Can you work these out from the model? Positions are in its coordinate system, mm. A direction names the side the tool comes from. Give positions to 0.01 mm unless a question says otherwise; leave off trailing zeros. Write each loop counter-clockwise with the first axis right and the second up, starting at its lowest first coordinate (ties: lowest second). Pieces come first, ordered by that corner, then holes.
Autodesk Inventor part; units mm, degrees
ref_plane "YZ Plane" through (0, 0, 0) normal (1, 0, 0) x (0, 1, 0)
ref_plane "XZ Plane" through (0, 0, 0) normal (0, 1, 0) x (-1, 0, 0)
ref_plane "XY Plane" through (0, 0, 0) normal (0, 0, 1) x (1, 0, 0)
sketch "Sketch1" plane through (0, 0, 0) normal (0, 1, 0) x (-1, 0, 0)
  circle A0 centre (0, 0) radius 13.3
  circle A1 centre (0, 0) radius 15.3
  dimension "d0" = 26.6
  dimension "d1" = 2
extrude "Extrusion1" add sketch "Sketch1" along normal blind 28 contours A0 | A1
sketch "Sketch2" plane through (0, 0, 0) normal (0, -1, 0) x (1, 0, 0)
  circle A0 centre (0, 0) radius 12
  circle A1 centre (0, 0) radius 14
  dimension "d4" = 24
  dimension "d5" = 2
extrude "Extrusion2" add sketch "Sketch2" along normal blind 30.55 contours A0 | A1
sketch "Sketch3" plane through (0, -30.55, 0) normal (0, -1, 0) x (1, 0, 0)
  circle A0 centre (0, 0) radius 3
  dimension "d8" = 6
extrude "Extrusion3" add sketch "Sketch3" along normal blind 2
sketch "Sketch4" plane through (0, 28, 0) normal (0, 1, 0) x (1, 0, 0)
  circle A0 centre (0, 0) radius 2
  dimension "d11" = 4
extrude "Extrusion4" add sketch "Sketch4" along normal blind 8.1
properties part number "Pump"
(1) Imagine slicing it at B-B, the plane z = 0. Write out the boundary of the cut face in (x, y), plus the area to 3 significant figures.
Returned:
outline: (-15.3, 0) - (-14, 0) - (-14, -30.55) - (-3, -30.55) - (-3, -32.55) - (3, -32.55) - (3, -30.55) - (14, -30.55) - (14, 0) - (15.3, 0) - (15.3, 28) - (2, 28) - (2, 36.1) - (-2, 36.1) - (-2, 28) - (-15.3, 28) - close
area: 1,760 mm2
(2) Imagine slicing it at D-D, the plane x = -13. Write out the boundary of the cut face in (y, z).
Returned:
outline: (-30.55, -5.2) - (0, -5.2) - (0, -8.07) - (28, -8.07) - (28, 8.07) - (0, 8.07) - (0, 5.2) - (-30.55, 5.2) - close
(3) Imagine slicing it at A-A, the plane x = 0. Write out the boundary of the cut face in (y, z).
Returned:
outline: (-32.55, -3) - (-30.55, -3) - (-30.55, -14) - (0, -14) - (0, -15.3) - (28, -15.3) - (28, -2) - (36.1, -2) - (36.1, 2) - (28, 2) - (28, 15.3) - (0, 15.3) - (0, 14) - (-30.55, 14) - (-30.55, 3) - (-32.55, 3) - close
(4) Will these pins go through, and if not, where does the flat tip stop? P1, Ø1, axis at x = -5.5, y = 13.5, coming from the +Z side; P2, Ø2, axis at x = -9.5, z = -4.5, coming from the +Y side; P3, Ø1, axis at y = 15.5, z = 2, coming from the +X side.
Returned:
P1: stops at z = 14.46
P2: stops at y = 28
P3: stops at x = 15.23
(5) Imagine slicing it at C-C, the plane y = -13.5. Write out the boundary of the cut face in (x, z), plus the area to 3 significant figures.
Returned:
outline: circle Ø28 at (0, 0)
area: 616 mm2
(6) If I drill on L1, parallel to Y at x = 8, z = -12; L2, parallel to Y at x = -3, z = -8.5; L3, parallel to X at y = -5, z = 11.5, over which ranges is the centre line in solid material (lowest first)?
Returned:
L1: y = 0 to 28
L2: y = -30.55 to 28
L3: x = -7.98 to 7.98
(7) For faces 1 (the face through (0, 32, -2)), 2 (the face through (0, -32.55, 0)), 3 (the face through (-14, 0, -4)), which set-ups out of +Z, -Z, +X, -X, +Y, -Y let a thin tool reach every point of the face, with its end or its side?
Returned:
face 1: +Y
face 2: +Z, -Z, +X, -X, -Y
face 3: -Y
